from build123d import *

# Parameters (mm, degrees)
SKETCH1_W           = 20
SKETCH1_H           = 10
BOSS_EXTRUDE1_DEPTH = 2
SKETCH2_W           = 10
SKETCH2_H           = 22
BOSS_EXTRUDE2_DEPTH = 2
FILLET1_R           = 2
FILLET2_R           = 1
SKETCH3_R           = 2
CUT_EXTRUDE1_DEPTH  = 2
SKETCH4_R           = 2
CUT_EXTRUDE2_DEPTH  = 2


with BuildPart() as part:
    # Sketch1 → Boss-Extrude1 (new body)
    with BuildSketch(Plane(origin=(0, 0, 0), x_dir=(1, 0, 0), z_dir=(0, 1, 0))):
        Rectangle(SKETCH1_W, SKETCH1_H)
    extrude(amount=BOSS_EXTRUDE1_DEPTH)

    # Sketch2 → Boss-Extrude2 (add)
    with BuildSketch(Plane.ZY.offset(10)):
        with Locations((0, 11)):
            Rectangle(SKETCH2_W, SKETCH2_H)
    extrude(amount=BOSS_EXTRUDE2_DEPTH)

    # Fillet1
    fillet1_edges = [part.edges().sort_by_distance(p)[0] for p in [
        (-12, 0, 0),
    ]]
    fillet(fillet1_edges, radius=FILLET1_R)

    # Fillet2
    fillet2_edges = [part.edges().sort_by_distance(p)[0] for p in [
        (-10, 2, 0),
    ]]
    fillet(fillet2_edges, radius=FILLET2_R)

    # Sketch3 → Cut-Extrude1 (cut)
    with BuildSketch(Plane(origin=(0, 2, 0), x_dir=(1, 0, 0), z_dir=(0, 1, 0))):
        with Locations(Location((-5, 0, 0), (0, 0, 270))):
            Circle(SKETCH3_R)
        with Locations(Location((5, 0, 0), (0, 0, 270))):
            Circle(SKETCH3_R)
    extrude(amount=-CUT_EXTRUDE1_DEPTH, mode=Mode.SUBTRACT)

    # Sketch4 → Cut-Extrude2 (cut)
    with BuildSketch(Plane(origin=(-10, 0, 0), x_dir=(0, 0, -1), z_dir=(1, 0, 0))):
        with Locations((0, 17)):
            Circle(SKETCH4_R)
        with Locations((0, 7)):
            Circle(SKETCH4_R)
    extrude(amount=-CUT_EXTRUDE2_DEPTH, mode=Mode.SUBTRACT)


solid = part.part
For this review, take the finished solid that the model builds, in its own axes (mm). A direction names the side the tool comes from. Round coordinates to 2 decimals unless told otherwise and drop trailing zeros. Loops run counter-clockwise (first coordinate to the right, second up) from the corner with the lowest first, then second, coordinate; pieces in that order, holes last. Notation, with made-up numbers: (1, -7) - (11, -7) arc R20 ccw to (11, 21) - close; hole circle Ø5 at (1, 36.5). An arc over 180 degrees is marked (long way). One line per question, with ' | ' between items.
Q1. For pin 1 (2.5 mm diameter, centred on x = 5, z = 0, fed in from +Y) (3 decimals); pin 2 (3 mm diameter, centred on x = 3.5, z = -1, fed in from +Y); pin 3 (3 mm diameter, centred on y = 12.5, z = -0.5, fed in from +X), all flat-tipped, find the tip position at first contact; note any pin that passes through.
Taken from the geometry:
pin 1: passes through | pin 2: stops at y = 2 | pin 3: stops at x = -10
Q2. For line 1 along Y through (x, z) = (-11.4, 0); line 2 along Y through (x, z) = (-10.7, 0); line 3 along X through (y, z) = (1.15, 0), list the stretches that pass through material, from the lowest coordinate up. Write a range as [from, to].
Taken from the geometry:
line 1: y = [0.57, 5], [9, 15], [19, 22] | line 2: y = [0.13, 5], [9, 15], [19, 22] | line 3: x = [-11.81, -7], [-3, 3], [7, 10]
Q3. Take a section at C-C (x = -5). Give the boundary of the cut face in (y, z), and give its area (3 significant figures).
Taken from the geometry:
outline: (0, -5) - (2, -5) - (2, -2) - (0, -2) - close; (0, 2) - (2, 2) - (2, 5) - (0, 5) - close | area: 12.0 mm²
Q4. Take a section at B-B (z = 0). Give the boundary of the cut face in (x, y), and give its area (3 significant figures).
Taken from the geometry:
outline: (-12, 2) arc R2 ccw to (-10, 0) - (-7, 0) - (-7, 2) - (-9, 2) arc R1 cw to (-10, 3) - (-10, 5) - (-12, 5) - close; (-12, 9) - (-10, 9) - (-10, 15) - (-12, 15) - close; (-12, 19) - (-10, 19) - (-10, 22) - (-12, 22) - close; (-3, 0) - (3, 0) - (3, 2) - (-3, 2) - close; (7, 0) - (10, 0) - (10, 2) - (7, 2) - close | area: 51.4 mm²
Q5. The part is to be moulded in two halves that separate along Y. For faces 3 (the flat face through (-10, 13, 0)), 4 (the cylindrical face through (-9.715, 2.301, -0.07)), 5 (the cylindrical face through (-11, 19, 0)), 6 (the cylindrical face through (-11, 9, 0)), say which applies: released by +Y, released by -Y, zero draft, split by the parting line, or undercut.
Taken from the geometry:
face 3: zero draft | face 4: released by +Y | face 5: undercut | face 6: undercut
Q6. Take a section at D-D (z = 2.5). Give the boundary of the cut face in (x, y).
Taken from the geometry:
outline: (-12, 2) arc R2 ccw to (-10, 0) - (10, 0) - (10, 2) - (-9, 2) arc R1 cw to (-10, 3) - (-10, 22) - (-12, 22) - close
Q7. Tool access review of faces 1 (the cylindrical face through (-11.4, 0.57, 0.07)), 2 (the flat face through (0, 2, 0)): name each direction out of +Z, -Z, +X, -X, +Y, -Y from which nothing blocks a thin tool from reaching the whole face with its end or side.
Taken from the geometry:
face 1: +Z, -Z, -X, -Y | face 2: +Z, -Z, +X, +Y
Q8. Take a section at A-A (y = 17). Give the boundary of the cut face in (x, z), and give its area (3 significant figures).
Taken from the geometry:
outline: (-12, -5) - (-10, -5) - (-10, -2) - (-12, -2) - close; (-12, 2) - (-10, 2) - (-10, 5) - (-12, 5) - close | area: 12.0 mm²
